Could you check a few things on this model? Use its own coordinates, in mm. Face numbers are marked on the shaded views. Give positions to 0.01 mm unless a question says otherwise; leave off trailing zeros. Loops run counter-clockwise (first coordinate to the right, second up) from the corner with the lowest first, then second, coordinate; pieces in that order, holes last. Notation, with made-up numbers: (80.25, 83.25) -> (94.25, 83.25) arc R21 cw to (94.25, 103.25) -> close; hole circle Ø1 at (33, -36). An arc over 180 degrees is marked (long way). Write item = value, one per line. Start each with the question number.
1) I want a section at B-B (x = 0). List the corners of the cut face in (y, z) for me, and give its area (4 significant figures).
2) I need wall thicknesses on probe 1 along Z at (x, y) = (0, 64); probe 2 along Z at (x, y) = (-117.5, 10.75). Which ranges of each line are inside material? Lowest first, please. Write a range as from..to.
3) I want a section at D-D (y = 43.5). List the corners of the cut face in (x, z) for me, and give its area (3 significant figures).
4) I'm going to push flat-ended pins straight in: pin 1 Ø20.5 at (x, z) = (-117.5, -50) entering from +Y; pin 2 Ø5 at (y, z) = (28, -27) entering from +X; pin 3 Ø2 at (y, z) = (32, -48) entering from -X; pin 4 Ø11 at (x, z) = (117.5, 50) entering from -Y. Where does each tip first touch, or does it pass through?
5) If we mould it in two halves opening along X, with no side actions, what happens to the marked faces 1, 2 and 3? For each: +X half, -X half, draft (parallel to the pull), parting line (faces both ways), or undercut.
6) I want a section at C-C (z = 55). List the corners of the cut face in (x, y) for me.
7) I want a section at A-A (z = 0). List the corners of the cut face in (x, y) for me, and give its area (3 significant figures).
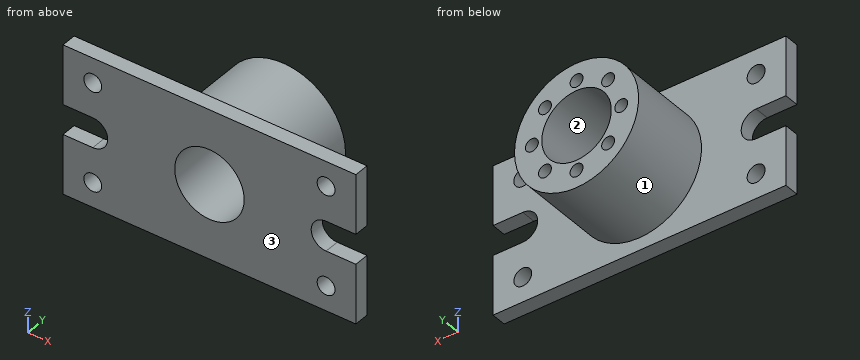
from build123d import *

# Parameters (mm, degrees)
SKETCH1_R           = 9
BOSS_EXTRUDE1_DEPTH = 15
SKETCH2_R           = 62.5
BOSS_EXTRUDE2_DEPTH = 85
SKETCH3_R           = 35
CUT_EXTRUDE1_DEPTH  = 101
SKETCH4_R           = 6.5
CUT_EXTRUDE2_DEPTH  = 50


with BuildPart() as part:
    # Sketch1 → Boss-Extrude1 (new body)
    with BuildSketch(Plane(origin=(0, 0, 0), x_dir=(1, 0, 0), z_dir=(0, 1, 0))):
        with BuildLine():
            Line((-147.5, -15), (-147.5, -75))
            Line((-147.5, -75), (147.5, -75))
            Line((147.5, -75), (147.5, -15))
            Line((147.5, -15), (117.5, -15))
            ThreePointArc((117.5, -15), (102.5, 0), (117.5, 15))
            Line((117.5, 15), (147.5, 15))
            Line((147.5, 15), (147.5, 75))
            Line((147.5, 75), (-147.5, 75))
            Line((-147.5, 75), (-147.5, 15))
            Line((-147.5, 15), (-117.5, 15))
            ThreePointArc((-117.5, 15), (-102.5, 0), (-117.5, -15))
            Line((-117.5, -15), (-147.5, -15))
        make_face()
        with Locations((-117.5, -50)):
            Circle(SKETCH1_R, mode=Mode.SUBTRACT)
        with Locations((117.5, -50)):
            Circle(SKETCH1_R, mode=Mode.SUBTRACT)
        with Locations((-117.5, 50)):
            Circle(SKETCH1_R, mode=Mode.SUBTRACT)
        with Locations((117.5, 50)):
            Circle(SKETCH1_R, mode=Mode.SUBTRACT)
    extrude(amount=BOSS_EXTRUDE1_DEPTH)

    # Sketch2 → Boss-Extrude2 (add)
    with BuildSketch(Plane(origin=(0, 15, 0), x_dir=(1, 0, 0), z_dir=(0, 1, 0))):
        Circle(SKETCH2_R)
    extrude(amount=BOSS_EXTRUDE2_DEPTH)

    # Sketch3 → Cut-Extrude1 (cut, through all)
    with BuildSketch(Plane(origin=(0, 100, 0), x_dir=(1, 0, 0), z_dir=(0, 1, 0))):
        Circle(SKETCH3_R)
    extrude(amount=-CUT_EXTRUDE1_DEPTH, mode=Mode.SUBTRACT)

    # Sketch4 → Cut-Extrude2 (cut)
    with BuildSketch(Plane(origin=(0, 100, 0), x_dir=(1, 0, 0), z_dir=(0, 1, 0))):
        with Locations((-45, 0)):
            Circle(SKETCH4_R)
        with Locations((-31.819805153, 31.819805153)):
            Circle(SKETCH4_R)
        with Locations((0, 45)):
            Circle(SKETCH4_R)
        with Locations((31.819805153, 31.819805153)):
            Circle(SKETCH4_R)
        with Locations((45, 0)):
            Circle(SKETCH4_R)
        with Locations((31.819805153, -31.819805153)):
            Circle(SKETCH4_R)
        with Locations((0, -45)):
            Circle(SKETCH4_R)
        with Locations((-31.819805153, -31.819805153)):
            Circle(SKETCH4_R)
    extrude(amount=-CUT_EXTRUDE2_DEPTH, mode=Mode.SUBTRACT)


solid = part.part
Answer list:
q1.outline = (0, -75) -> (15, -75) -> (15, -62.5) -> (100, -62.5) -> (100, -51.5) -> (50, -51.5) -> (50, -38.5) -> (100, -38.5) -> (100, -35) -> (0, -35) -> close; (0, 35) -> (100, 35) -> (100, 38.5) -> (50, 38.5) -> (50, 51.5) -> (100, 51.5) -> (100, 62.5) -> (15, 62.5) -> (15, 75) -> (0, 75) -> close
q1.area = 4,575 mm^2
q2.probe_1 = -62.5..-51.5, -38.5..-35, 35..38.5, 51.5..62.5
q2.probe_2 = -75..-59, -41..-15, 15..41, 59..75
q3.outline = circle Ø125 at (0, 0); hole circle Ø70 at (0, 0)
q3.area = 8,420 mm^2
q4.pin_1 = 15
q4.pin_2 = 57.5
q4.pin_3 = -41.2
q4.pin_4 = through
q5.face_1 = parting line
q5.face_2 = undercut
q5.face_3 = draft
q6.outline = (-147.5, 0) -> (-124.98, 0) -> (-124.98, 15) -> (-147.5, 15) -> close; (-110.02, 0) -> (110.02, 0) -> (110.02, 15) -> (29.69, 15) -> (29.69, 100) -> (-29.69, 100) -> (-29.69, 15) -> (-110.02, 15) -> close; (124.98, 0) -> (147.5, 0) -> (147.5, 15) -> (124.98, 15) -> close
q7.outline = (-102.5, 0) -> (-35, 0) -> (-35, 100) -> (-38.5, 100) -> (-38.5, 50) -> (-51.5, 50) -> (-51.5, 100) -> (-62.5, 100) -> (-62.5, 15) -> (-102.5, 15) -> close; (35, 0) -> (102.5, 0) -> (102.5, 15) -> (62.5, 15) -> (62.5, 100) -> (51.5, 100) -> (51.5, 50) -> (38.5, 50) -> (38.5, 100) -> (35, 100) -> close
q7.area = 5,400 mm^2
